Drawing for the job (mm, zero at the part's lowest x, y, z). A direction names the side the tool comes from. Give positions to 0.01 mm unless a question says otherwise; leave off trailing zeros. Loops run counter-clockwise (first coordinate to the right, second up) from the corner with the lowest first, then second, coordinate; pieces in that order, holes last. Notation, with made-up numbers: (-12.75, -7) -> (11.25, -7) arc R25 ccw to (11.25, 11) -> close; hole circle Ø10 at (59, 76). An arc over 180 degrees is marked (long way). Write item = value, one per line.
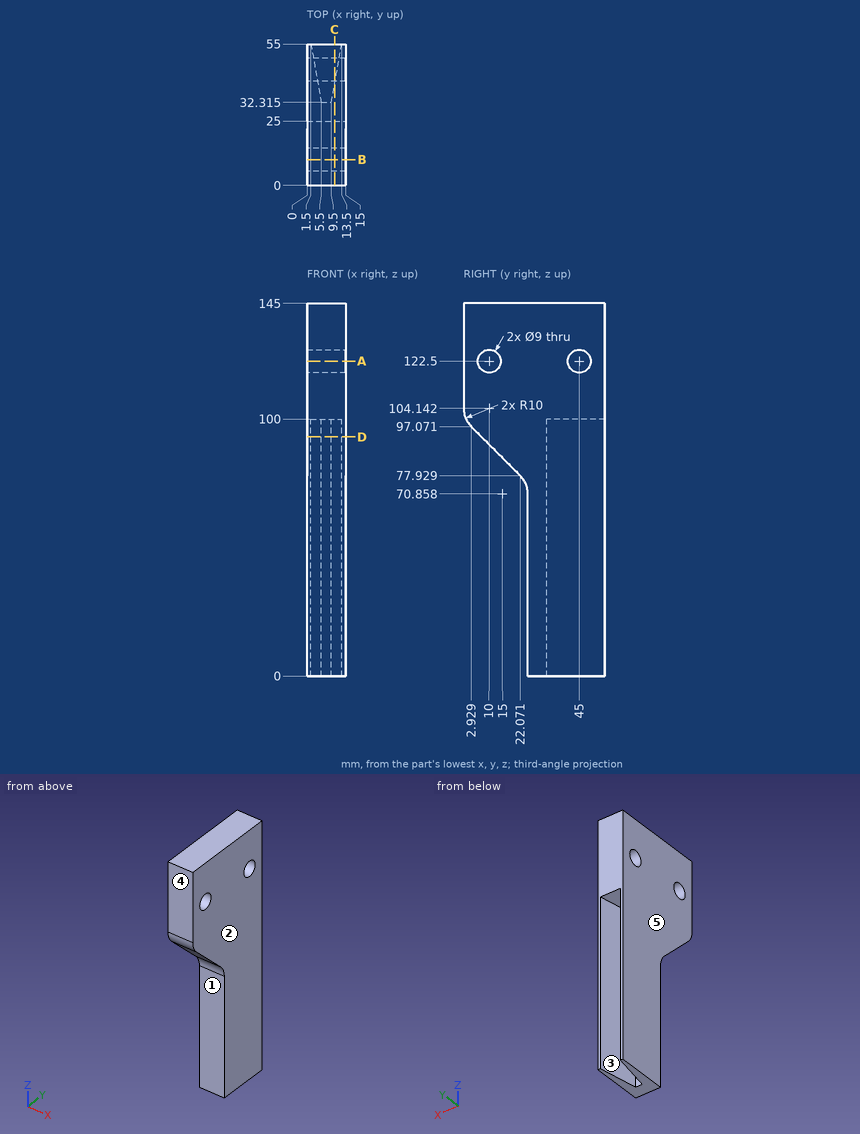
1) Drill centre lines: line 1 along Y through (x, z) = (8, 122.5); line 2 along Y through (x, z) = (7.75, 126.5); line 3 along Z through (x, y) = (9.5, 46.5). Where is each one in solid material? Low to high. Write a range as [from, to].
Resolved:
line_1 = [0, 5.5], [14.5, 40.5], [49.5, 55]
line_2 = [0, 7.94], [12.06, 42.94], [47.06, 55]
line_3 = [100, 118.26], [126.74, 145]
2) Slice it at C-C, the plane x = 10.75. List the corners of the cut face in (y, z), and give its area (3 significant figures).
Resolved:
outline = (0, 104.14) arc R10 ccw to (2.93, 97.07) -> (22.07, 77.93) arc R10 cw to (25, 70.86) -> (25, 0) -> (39.4, 0) -> (39.4, 100) -> (55, 100) -> (55, 145) -> (0, 145) -> close; hole circle Ø9 at (10, 122.5); hole circle Ø9 at (45, 122.5)
area = 4,100 mm²
3) Slice it at D-D, the plane z = 93. List the corners of the cut face in (x, y) (3 decimals).
Resolved:
outline = (0, 7) -> (15, 7) -> (15, 55) -> (13.5, 55) -> (9.5, 32.315) -> (5.5, 32.315) -> (1.5, 55) -> (0, 55) -> close
4) Slice it at A-A, the plane z = 122.5. List the corners of the cut face in (x, y), and give its area (3 significant figures).
Resolved:
outline = (0, 0) -> (15, 0) -> (15, 5.5) -> (0, 5.5) -> close; (0, 14.5) -> (15, 14.5) -> (15, 40.5) -> (0, 40.5) -> close; (0, 49.5) -> (15, 49.5) -> (15, 55) -> (0, 55) -> close
area = 555 mm²
5) Pull direction X, two halves, no side cores. Call the marked faces 3, 4 and 5: pulls with the +X half, pulls with the -X half, needs draft (parallel to the pull), parting line crosses it, or undercut.
Resolved:
face_3 = undercut
face_4 = needs draft
face_5 = pulls with the -X half
6) Which spindle directions (+Z, -Z, +X, -X, +Y, -Y) get a long thin tool onto all of the face, cutting with end or side? Do the marked faces 1 and 2. Say none if no direction does.
Resolved:
face_1 = -Z, +X, -X, -Y
face_2 = +Z, -Z, +X, +Y, -Y
7) Slice it at B-B, the plane y = 10. List the corners of the cut face in (x, z), and give its area (3 significant figures).
Resolved:
outline = (0, 90) -> (15, 90) -> (15, 118) -> (0, 118) -> close; (0, 127) -> (15, 127) -> (15, 145) -> (0, 145) -> close
area = 690 mm²
8) Drop flat-ended pins along their axis: P1, Ø2, axis at x = 13, y = 22, coming from the -Z side; P2, Ø4.5, axis at x = 6.5, z = 31, coming from the -Y side; P3, Ø1.2, axis at x = 7.5, z = 37.5, coming from the +Y side (3 decimals). Give the stop position or say it passes through.
Resolved:
P1 = 76.86
P2 = 25
P3 = 32.315
